```python
from build123d import *

# Parameters (mm, degrees)
SKETCH1_R           = 125
BOSS_EXTRUDE1_DEPTH = 75
FILLET1_R           = 30
SKETCH2_R           = 50
CUT_EXTRUDE1_DEPTH  = 20
SKETCH3_R           = 30
CUT_EXTRUDE2_DEPTH  = 50


with BuildPart() as part:
    # Sketch1 → Boss-Extrude1 (new, symmetric)
    with BuildSketch(Plane(origin=(0, 0, 0), x_dir=(0, 0, -1), z_dir=(1, 0, 0))):
        Circle(SKETCH1_R)
    extrude(amount=BOSS_EXTRUDE1_DEPTH, both=True)

    # Fillet1
    fillet1_edges = [part.edges().sort_by_distance(p)[0] for p in [
        (-75, 0, 125),
        (75, 0, 125),
    ]]
    fillet(fillet1_edges, radius=FILLET1_R)

    # Sketch2 → Cut-Extrude1 (cut)
    with BuildSketch(Plane(origin=(75, 0, 0), x_dir=(0, 0, -1), z_dir=(1, 0, 0))):
        Circle(SKETCH2_R)
    extrude(amount=-CUT_EXTRUDE1_DEPTH, mode=Mode.SUBTRACT)

    # Sketch3 → Cut-Extrude2 (cut)
    with BuildSketch(Plane.ZY.offset(75)):
        Circle(SKETCH3_R)
    extrude(amount=-CUT_EXTRUDE2_DEPTH, mode=Mode.SUBTRACT)


solid = part.part
```
Part model, mm, in its own coordinate system. A direction names the side the tool comes from. Give positions to 0.01 mm unless a question says otherwise; leave off trailing zeros. Order: outer loops, then holes, each group sorted by start corner. A loop starts at its lowest first (then second) coordinate and runs counter-clockwise, first axis right, second up. Notation, with made-up numbers: M 20,34 L 62,34 A26 ccw 62,73 Z; hole C 48,79.25 d5. An arc over 180 degrees is marked long. Use a Markdown table: item, result. Add a question column.
(1) 3-axis set-ups, long thin cutter, end or side, ignore diameter. For faces 1 (the face through (65.14, 15.02, -47.69)), 2 (the face through (-75, 22, 22)), 3 (the face through (-25, 0, 0)): which of +Z, -Z, +X, -X, +Y, -Y reach the whole face in a straight line?
(2) Probe line 1 along Z through (x, y) = (56, 15.5); line 2 along X through (y, z) = (1, -42); line 3 along Y through (x, z) = (-56, 0). List the from-to ranges inside material, lowest first. Write a range as [from, to].
(3) Drop flat-ended pins along their axis: P1, Ø2, axis at x = -44.5, y = 71.5, coming from the +Z side; P2, Ø8, axis at x = -14.5, y = -20, coming from the -Z side; P3, Ø1, axis at x = 38, z = -65.5, coming from the -Y side. Give the stop position or say it passes through.
(4) Saw through at D-D, the plane x = 58.5. Give the cut face in (y, z), and give its area (3 significant figures).
(5) Saw through at A-A, the plane y = 0. Give the cut face in (x, z), and give its area (3 significant figures).
(6) Saw through at C-C, the plane x = 5. Give the cut face in (y, z).
(7) Mould opens along Z. For faces 4 (the face through (-50.35, 1.32, -29.97)), 5 (the face through (0.63, 5.5, 124.88)), 6 (the face through (75, -41, -41)), 7 (the face through (55, 1, 1)) say: +Z half, -Z half, draft (parallel to the pull), parting line (faces both ways), or undercut.
Answer key:
| question | item | result |
|---|---|---|
| 1 | face 1 | +X |
| 1 | face 2 | +Z, -Z, -X, +Y, -Y |
| 1 | face 3 | -X |
| 2 | line 1 | [-121.93, -47.54], [47.54, 121.93] |
| 2 | line 2 | [-75, 55] |
| 2 | line 3 | [-122.91, -30], [30, 122.91] |
| 3 | P1 | z = 103.22 |
| 3 | P2 | z = -123.97 |
| 3 | P3 | y = -106.77 |
| 4 | outline | C 0,0 d243.58; hole C 0,0 d100 |
| 4 | area | 38,700 mm^2 |
| 5 | outline | M -75,-95 A30 ccw -45,-125 L 45,-125 A30 ccw 75,-95 L 75,-50 L 55,-50 L 55,50 L 75,50 L 75,95 A30 ccw 45,125 L -45,125 A30 ccw -75,95 L -75,30 L -25,30 L -25,-30 L -75,-30 Z |
| 5 | area | 31,700 mm^2 |
| 6 | outline | C 0,0 d250 |
| 7 | face 4 | undercut |
| 7 | face 5 | parting line |
| 7 | face 6 | draft |
| 7 | face 7 | undercut |
